from build123d import *

# Parameters (mm, degrees)
SKETCH1_W          = 1.6
SKETCH1_H          = 10.2
BASE_FLANGE1_DEPTH = 1.5


# Sheet-metal steps are written as plain solids
with BuildPart() as part:
    # Sketch1 → Base-Flange1 (new body)
    with BuildSketch(Plane.XY):
        with BuildLine():
            Line((0.2, 0), (45.05, 0))
            ThreePointArc((45.05, 0), (45.191421356, 0.058578644), (45.25, 0.2))
            Line((45.25, 0.2), (45.25, 15.8))
            ThreePointArc((45.25, 15.8), (45.191421356, 15.941421356), (45.05, 16))
            Line((45.05, 16), (0.2, 16))
            ThreePointArc((0.2, 16), (0.058578644, 15.941421356), (0, 15.8))
            Line((0, 15.8), (0, 0.2))
            ThreePointArc((0, 0.2), (0.058578644, 0.058578644), (0.2, 0))
        make_face()
        with Locations((3.172093023, 8)):
            Rectangle(SKETCH1_W, SKETCH1_H, mode=Mode.SUBTRACT)
        with Locations((42.077906977, 8)):
            Rectangle(SKETCH1_W, SKETCH1_H, mode=Mode.SUBTRACT)
    extrude(amount=-BASE_FLANGE1_DEPTH)


solid = part.part
Geometry: final body of the model. Coordinates: model frame, mm. A direction names the side the tool comes from. Coordinates: 2 decimals unless noted, no trailing zeros. Write each loop counter-clockwise with the first axis right and the second up, starting at its lowest first coordinate (ties: lowest second). Pieces come first, ordered by that corner, then holes. Notation, with made-up numbers: (-10, -33.75) - (46, -33.75) arc R23 ccw to (46, -12.75) - close; hole circle Ø3 at (-11.5, -10). An arc over 180 degrees is marked (long way). Return JSON: item names as keys, results as strings.
Item 1: Section query B-B (z = -0.5). Output: boundary loops of the cut face in (x, y), and give its area (3 significant figures).
Completed:
{"outline": "(0, 0.2) arc R0.2 ccw to (0.2, 0) - (45.05, 0) arc R0.2 ccw to (45.25, 0.2) - (45.25, 15.8) arc R0.2 ccw to (45.05, 16) - (0.2, 16) arc R0.2 ccw to (0, 15.8) - close; hole (2.37, 2.9) - (3.97, 2.9) - (3.97, 13.1) - (2.37, 13.1) - close; hole (41.28, 2.9) - (42.88, 2.9) - (42.88, 13.1) - (41.28, 13.1) - close", "area": "691 mm2"}
Item 2: Line query: L1, parallel to X at y = 4.5, z = -0.8. Output: solid intervals per line, ascending.
Completed:
{"L1": "x = 0 to 2.37, 3.97 to 41.28, 42.88 to 45.25"}
Item 3: Section query A-A (y = 3.5). Output: boundary loops of the cut face in (x, z), and give its area (3 significant figures).
Completed:
{"outline": "(0, -1.5) - (2.37, -1.5) - (2.37, 0) - (0, 0) - close; (3.97, -1.5) - (41.28, -1.5) - (41.28, 0) - (3.97, 0) - close; (42.88, -1.5) - (45.25, -1.5) - (45.25, 0) - (42.88, 0) - close", "area": "63.1 mm2"}
Item 4: Reachability of faces 1 (the face through (2.372, 8, -1)), 2 (the face through (45.25, 8, -1)) from +Z, -Z, +X, -X, +Y, -Y: full face, straight path, thin tool, end or side. Return the list, or none.
Completed:
{"face 1": "+Z, -Z", "face 2": "+Z, -Z, +X, +Y, -Y"}
Item 5: Pull-direction query (Y, two-part tool) for faces 3 (the face through (22, 8, -1.5)), 4 (the face through (41.278, 8, -1)), 5 (the face through (22, 0, -1)); classes: +Y half, -Y half, draft (parallel to the pull), parting line (faces both ways), or undercut.
Completed:
{"face 3": "draft", "face 4": "undercut", "face 5": "-Y half"}
